from build123d import *

# Parameters (mm, degrees)
SKETCH_1_R          = 9.5
SKETCH_1_R_2        = 2.5
EXTRUDE_1_DEPTH     = 24.5
CHAMFER_1_SIZE      = 0.5
SKETCH_2_R          = 4
CUT_EXTRUDE_1_DEPTH = 10
SKETCH_3_R          = 1.5
CUT_EXTRUDE_2_DEPTH = 10


with BuildPart() as part:
    # 草图1 → 凸台-拉伸1 (new body)
    with BuildSketch(Plane(origin=(0, 0, 0), x_dir=(1, 0, 0), z_dir=(0, 1, 0))):
        with Locations(Location((0, 0, 0), (0, 0, 270))):
            Circle(SKETCH_1_R)
        with Locations(Location((0, 0, 0), (0, 0, 270))):
            Circle(SKETCH_1_R_2, mode=Mode.SUBTRACT)
    extrude(amount=EXTRUDE_1_DEPTH)

    # 倒角1
    chamfer_1_edges = [part.edges().sort_by_distance(p)[0] for p in [
        (0, 0, -9.5),
        (0, 24.5, -9.5),
    ]]
    chamfer(chamfer_1_edges, length=CHAMFER_1_SIZE)

    # 草图2 → 切除-拉伸1 (cut)
    with BuildSketch(Plane.XZ):
        with Locations(Location((0, 0, 0), (0, 0, 270))):
            Circle(SKETCH_2_R)
    extrude(amount=-CUT_EXTRUDE_1_DEPTH, mode=Mode.SUBTRACT)

    # 草图3 → 切除-拉伸2 (cut)
    with BuildSketch(Plane.XY.offset(9.5)):
        with Locations((0, 6)):
            Circle(SKETCH_3_R)
        with Locations((0, 18.5)):
            Circle(SKETCH_3_R)
    extrude(amount=-CUT_EXTRUDE_2_DEPTH, mode=Mode.SUBTRACT)


solid = part.part
Can you work these out from the model? Positions are in its coordinate system, mm. A direction names the side the tool comes from. Give positions to 0.01 mm unless a question says otherwise; leave off trailing zeros. Loops run counter-clockwise (first coordinate to the right, second up) from the corner with the lowest first, then second, coordinate; pieces in that order, holes last. Notation, with made-up numbers: (76.25, -40) - (126.25, -40) arc R16 ccw to (126.25, -28) - close; hole circle Ø5 at (50, 10). An arc over 180 degrees is marked (long way). Answer as a JSON object with one key per item and string values.
Q1. Imagine slicing it at B-B on x = 0. Write out the boundary of the cut face in (y, z), plus the area to 3 significant figures.
Geometry says:
{"outline": "(0, -9) - (0.5, -9.5) - (24, -9.5) - (24.5, -9) - (24.5, -2.5) - (10, -2.5) - (10, -4) - (0, -4) - close; (0, 4) - (4.5, 4) - (4.5, 9.5) - (0.5, 9.5) - (0, 9) - close; (7.5, 4) - (10, 4) - (10, 2.5) - (17, 2.5) - (17, 9.5) - (7.5, 9.5) - close; (20, 2.5) - (24.5, 2.5) - (24.5, 9) - (24, 9.5) - (20, 9.5) - close", "area": "275 mm²"}
Q2. If I drill on L1, parallel to Y at x = 0, z = 5.25; L2, parallel to Y at x = -0.5, z = 4.5; L3, parallel to X at y = 15.5, z = 0, over which ranges is the centre line in solid material (lowest first)?
Geometry says:
{"L1": "0 to 4.5, 7.5 to 17, 20 to 24.5", "L2": "0 to 4.59, 7.41 to 17.09, 19.91 to 24.5", "L3": "-9.5 to -2.5, 2.5 to 9.5"}
Q3. Imagine slicing it at D-D on y = 6.5. Write out the boundary of the cut face in (x, z).
Geometry says:
{"outline": "(-1.41, 3.74) - (-1.41, 9.39) arc R9.5 ccw (long way) to (1.41, 9.39) - (1.41, 3.74) arc R4 cw (long way) to start"}
Q4. Which directions (+Z, -Z, +X, -X, +Y, -Y) give clear straight access to the entire face, cutting with the end or side of a thin tool? Please do faces 5 (the flat face through (-2, 0, 4)), 6 (the cylindrical face through (-0.325, 4.536, 6.645)).
Geometry says:
{"face 5": "+Z, -Z, +X, -X, -Y", "face 6": "+Z"}
Q5. Imagine slicing it at A-A on z = 0. Write out the boundary of the cut face in (x, y).
Geometry says:
{"outline": "(-9.5, 0.5) - (-9, 0) - (-4, 0) - (-4, 10) - (-2.5, 10) - (-2.5, 24.5) - (-9, 24.5) - (-9.5, 24) - close; (2.5, 10) - (4, 10) - (4, 0) - (9, 0) - (9.5, 0.5) - (9.5, 24) - (9, 24.5) - (2.5, 24.5) - close"}
Q6. Will these pins go through, and if not, where does the flat tip stop? P1, Ø6, axis at y = 12, z = 0.5, coming from the -X side; P2, Ø4, axis at x = -1.5, z = -0.5, coming from the -Y side; P3, Ø1.5, axis at y = 17, z = -2, coming from the -X side; P4, Ø1, axis at x = 0.5, y = 6.5, coming from the +Z side.
Geometry says:
{"P1": "x = -9.5", "P2": "y = 10", "P3": "x = -9.42", "P4": "z = -3.87"}
Q7. Imagine slicing it at C-C on y = 9.25. Write out the boundary of the cut face in (x, z), plus the area to 3 significant figures.
Geometry says:
{"outline": "circle Ø19 at (0, 0); hole circle Ø8 at (0, 0)", "area": "233 mm²"}
Q8. If we mould it in two halves opening along Z, with no side actions, what happens to faces 1 (the flat face through (-2, 24.5, 2)), 2 (the flat face through (2, 10, -2)), 3 (the cylindrical face through (-5.78, 12.09, -7.54)), 4 (the cylindrical face through (-1.532, 4.93, -3.695))? For each: pulls with the +Z half, pulls with the -Z half, needs draft (parallel to the pull), parting line crosses it, or undercut.
Geometry says:
{"face 1": "needs draft", "face 2": "undercut", "face 3": "parting line crosses it", "face 4": "undercut"}
